Could you check a few things on this model? Use its own coordinates, in mm. A direction names the side the tool comes from. Round coordinates to 2 decimals unless told otherwise and drop trailing zeros. Order: outer loops, then holes, each group sorted by start corner. A loop starts at its lowest first (then second) coordinate and runs counter-clockwise, first axis right, second up. Notation, with made-up numbers: (47, 41.5) - (82, 41.5) arc R6 cw to (82, 48.5) - close; hole circle Ø7 at (9, -17.5). An arc over 180 degrees is marked (long way). Use one line per item in the form item = value.
from build123d import *

# Parameters (mm, degrees)
F0_R     = 2.5
F1_DEPTH = 12
F2_DEPTH = 12
F0_R_2   = 4
F3_DEPTH = 4
F4_DEPTH = 4
F5_R     = 1
F6_R     = 2
F7_DEPTH = 4.2
F8_DEPTH = 2.8


with BuildPart() as f1:
    # F0 (on Top) → F1 (new body)
    with BuildSketch(Plane.XY):
        Circle(F0_R)
    extrude(amount=F1_DEPTH)

    # F0 (on Top) → F2 (join)
    with BuildSketch(Plane.XY):
        Circle(F0_R)
    extrude(amount=-F2_DEPTH)

    # F0 (on Top) → F3 (join)
    with BuildSketch(Plane.XY):
        Circle(F0_R_2)
        Circle(F0_R, mode=Mode.SUBTRACT)
    extrude(amount=F3_DEPTH)

    # F0 (on Top) → F4 (join)
    with BuildSketch(Plane.XY):
        Circle(F0_R_2)
        Circle(F0_R, mode=Mode.SUBTRACT)
    extrude(amount=-F4_DEPTH)

    # F5
    f5_edges = [f1.edges().sort_by_distance(p)[0] for p in [
        (-2.5, 0, 12),
        (-2.5, 0, -12),
    ]]
    fillet(f5_edges, radius=F5_R)

    # F6 (on Front) → F7 (cut)
    with BuildSketch(Plane.XZ):
        Circle(F6_R)
    extrude(amount=-F7_DEPTH, mode=Mode.SUBTRACT)

    # F6 (on Front) → F8 (cut)
    with BuildSketch(Plane.XZ):
        Circle(F6_R)
    extrude(amount=F8_DEPTH, mode=Mode.SUBTRACT)


solid = f1.part
Item 1: For faces 4 (the face through (-0.54, -2.44, -7.45)), 5 (the face through (2, 2, 4)), 6 (the face through (0, 0, 12)), which set-ups out of +Z, -Z, +X, -X, +Y, -Y let a thin tool reach every point of the face, with its end or its side?
Found:
face_4 = -Z
face_5 = +Z
face_6 = +Z, +X, -X, +Y, -Y
Item 2: Imagine slicing it at B-B on z = 3. Please give me the cut outline in (x, y), plus the area to 3 significant figures.
Found:
outline = circle Ø8 at (0, 0)
area = 50.3 mm2
Item 3: Imagine slicing it at A-A on x = 0. Please give me the cut outline in (y, z), plus the area to 3 significant figures.
Found:
outline = (-4, -4) - (-2.5, -4) - (-2.5, -11) arc R1 ccw to (-1.5, -12) - (1.5, -12) arc R1 ccw to (2.5, -11) - (2.5, -4) - (4, -4) - (4, -2) - (-2.8, -2) - (-2.8, 2) - (4, 2) - (4, 4) - (2.5, 4) - (2.5, 11) arc R1 ccw to (1.5, 12) - (-1.5, 12) arc R1 ccw to (-2.5, 11) - (-2.5, 4) - (-4, 4) - close
area = 116 mm2
Item 4: Will these pins go through, and if not, where does the flat tip stop? P1, Ø1.2, axis at x = 0.5, z = 0.5, coming from the +Y side; P2, Ø1.5, axis at x = -3, z = -1, coming from the -Y side; P3, Ø1, axis at x = 2, y = 1.5, coming from the +Z side.
Found:
P1 = -2.8
P2 = -3.31
P3 = 11.87
Item 5: If we mould it in two halves opening along X, with no side actions, what happens to faces 1 (the face through (-0.54, -2.44, 7.55)), 2 (the face through (0, -2.8, 0)), 3 (the face through (2, 2, -4))? For each: released by +X, released by -X, zero draft, split by the parting line, or undercut.
Found:
face_1 = split by the parting line
face_2 = undercut
face_3 = zero draft
Item 6: Imagine slicing it at D-D on z = 0. Please give me the cut outline in (x, y), plus the area to 3 significant figures.
Found:
outline = (-2, -2.8) - (-2, 3.46) arc R4 ccw (long way) to (2, 3.46) - (2, -2.8) - close
area = 23.8 mm2
Item 7: I need wall thicknesses on L1, parallel to Z at x = 0, y = 3.05; L2, parallel to Z at x = 0, y = 1.4; L3, parallel to Y at x = 2, z = 5.25. Which ranges of each line are inside material? Lowest first, please.
Found:
L1 = -4 to -2, 2 to 4
L2 = -12 to -2, 2 to 12
L3 = -1.5 to 1.5
Item 8: Imagine slicing it at C-C on z = -4.25. Please give me the cut outline in (x, y).
Found:
outline = circle Ø5 at (0, 0)
